```python
from build123d import *

# Parameters (mm, degrees)
SKETCH_3_W             = 131
SKETCH_3_H             = 80
EXTRUDE_3_DEPTH        = 5
SKETCH_4_W             = 119
SKETCH_4_H             = 80
EXTRUDE_4_DEPTH        = 6
FILLET_2_R             = 5
CHAMFER_1_SIZE         = 1
CUT_EXTRUDE_1_DEPTH    = 6
FILLET_3_R             = 5
CHAMFER_2_SIZE         = 1
SKETCH_6_R             = 2.2
CUT_EXTRUDE_2_DEPTH    = 11
HOLE_WIZARD_M3_1_D     = 2.5
HOLE_WIZARD_M3_1_DEPTH = 7.5
HOLE_WIZARD_M3_1_TIP   = 0.751075774
CHAMFER_3_SIZE         = 0.5


with BuildPart() as part:
    # 草图3 → 凸台-拉伸3 (new body)
    with BuildSketch(Plane.XY):
        with Locations((0, -51.5)):
            Rectangle(SKETCH_3_W, SKETCH_3_H)
    extrude(amount=EXTRUDE_3_DEPTH)

    # 草图4 → 凸台-拉伸4 (add)
    with BuildSketch(Plane.XY.offset(5)):
        with Locations((0, -51.5)):
            Rectangle(SKETCH_4_W, SKETCH_4_H)
    extrude(amount=-EXTRUDE_4_DEPTH)

    # 圆角2
    fillet_2_edges = [part.edges().sort_by_distance(p)[0] for p in [
        (-65.5, -11.5, 2.5),
        (65.5, -11.5, 2.5),
        (65.5, -91.5, 2.5),
        (-65.5, -91.5, 2.5),
    ]]
    fillet(fillet_2_edges, radius=FILLET_2_R)

    # 倒角1
    chamfer_1_edges = [part.edges().sort_by_distance(p)[0] for p in [
        (0, -11.5, 5),
        (65.5, -51.5, 5),
        (0, -91.5, 5),
        (-65.5, -51.5, 5),
        (64.035533906, -90.035533906, 5),
        (-64.035533906, -90.035533906, 5),
        (-64.035533906, -12.964466094, 5),
        (64.035533906, -12.964466094, 5),
    ]]
    chamfer(chamfer_1_edges, length=CHAMFER_1_SIZE)

    # 草图5 → 切除-拉伸1 (cut)
    with BuildSketch(Plane.XY.offset(5)):
        Polygon((-10.644021059, -51.5), (-54.5, -28.163791023), (-54.5, -74.836208978), align=None)
        Polygon((43.855978941, -22.5), (-43.855978941, -22.5), (0, -45.836208978), align=None)
        Polygon((54.5, -28.163791023), (10.644021059, -51.5), (54.5, -74.836208978), align=None)
        Polygon((43.855978941, -80.5), (0, -57.163791023), (-43.855978941, -80.5), align=None)
    extrude(amount=-CUT_EXTRUDE_1_DEPTH, mode=Mode.SUBTRACT)

    # 圆角3
    fillet_3_edges = [part.edges().sort_by_distance(p)[0] for p in [
        (10.644021059, -51.5, 2),
        (54.5, -28.163791023, 2),
        (54.5, -74.836208978, 2),
        (-43.855978941, -22.5, 2),
        (43.855978941, -22.5, 2),
        (0, -45.836208978, 2),
        (-43.855978941, -80.5, 2),
        (0, -57.163791023, 2),
        (43.855978941, -80.5, 2),
        (-54.5, -74.836208978, 2),
        (-54.5, -28.163791023, 2),
        (-10.644021059, -51.5, 2),
    ]]
    fillet(fillet_3_edges, radius=FILLET_3_R)

    # 倒角2
    chamfer_2_edges = [part.edges().sort_by_distance(p)[0] for p in [
        (33.045284631, -39.580061586, 5),
        (54.5, -51.5, 5),
        (33.045284631, -63.419938415, 5),
        (14.256439507, -38.250213644, 5),
        (-14.256439507, -38.250213644, 5),
        (0, -22.5, 5),
        (-33.045284631, -39.580061586, 5),
        (-33.045284631, -63.419938415, 5),
        (-54.5, -51.5, 5),
        (-14.256439507, -64.749786356, 5),
        (14.256439507, -64.749786356, 5),
        (0, -80.5, 5),
        (52.074521107, -32.201893935, 5),
        (52.074521107, -70.798106066, 5),
        (16.288042118, -51.5, 5),
        (0, -45.172417956, 5),
        (-28.666695849, -26.289632976, 5),
        (28.666695849, -26.289632976, 5),
        (-16.288042118, -51.5, 5),
        (-52.074521107, -70.798106066, 5),
        (-52.074521107, -32.201893935, 5),
        (0, -57.827582045, 5),
        (28.666695849, -76.710367025, 5),
        (-28.666695849, -76.710367025, 5),
    ]]
    chamfer(chamfer_2_edges, length=CHAMFER_2_SIZE)

    # 草图6 → 切除-拉伸2 (cut)
    with BuildSketch(Plane.XY.offset(5)):
        with Locations((62.5, -21.5)):
            Circle(SKETCH_6_R)
        with Locations((62.5, -31.5)):
            Circle(SKETCH_6_R)
        with Locations((62.5, -41.5)):
            Circle(SKETCH_6_R)
        with Locations((62.5, -51.5)):
            Circle(SKETCH_6_R)
        with Locations((62.5, -61.5)):
            Circle(SKETCH_6_R)
        with Locations((62.5, -71.5)):
            Circle(SKETCH_6_R)
        with Locations((62.5, -81.5)):
            Circle(SKETCH_6_R)
    cut_extrude_2 = extrude(amount=-CUT_EXTRUDE_2_DEPTH, mode=Mode.SUBTRACT)

    # 镜向1: 切除-拉伸2 across plane
    add(cut_extrude_2.mirror(Plane(origin=(0, 0, 0), x_dir=(0, 0, 1), z_dir=(1, 0, 0))), mode=Mode.SUBTRACT)

    # M3 螺纹孔1
    with Locations(Plane.XY.offset(5)):
        with Locations((-43.51, -20.75), (43.51, -20.75), (43.51, -80.29), (-43.51, -80.29)):
            Hole(HOLE_WIZARD_M3_1_D / 2, depth=HOLE_WIZARD_M3_1_DEPTH)
            with Locations((0, 0, -(HOLE_WIZARD_M3_1_DEPTH + HOLE_WIZARD_M3_1_TIP / 2))):  # 118° drill point
                Cone(0, HOLE_WIZARD_M3_1_D / 2, HOLE_WIZARD_M3_1_TIP, mode=Mode.SUBTRACT)

    # 倒角3
    chamfer_3_edges = [part.edges().sort_by_distance(p)[0] for p in [
        (33.045284631, -39.580061586, -1),
        (54.5, -51.5, -1),
        (33.045284631, -63.419938415, -1),
        (14.256439507, -38.250213644, -1),
        (-60, -11.5, 0),
        (-14.256439507, -38.250213644, -1),
        (0, -22.5, -1),
        (60, -91.5, 0),
        (-33.045284631, -39.580061586, -1),
        (-33.045284631, -63.419938415, -1),
        (-54.5, -51.5, -1),
        (-14.256439507, -64.749786356, -1),
        (14.256439507, -64.749786356, -1),
        (0, -80.5, -1),
        (52.074521107, -32.201893935, -1),
        (52.074521107, -70.798106066, -1),
        (16.288042118, -51.5, -1),
        (0, -45.172417956, -1),
        (-28.666695849, -26.289632976, -1),
        (28.666695849, -26.289632976, -1),
        (-16.288042118, -51.5, -1),
        (-52.074521107, -70.798106066, -1),
        (-52.074521107, -32.201893935, -1),
        (0, -57.827582045, -1),
        (28.666695849, -76.710367025, -1),
        (-28.666695849, -76.710367025, -1),
        (0, -91.5, -1),
        (0, -11.5, -1),
        (60, -11.5, 0),
        (65.5, -51.5, 0),
        (64.035533906, -90.035533906, 0),
        (64.035533906, -12.964466094, 0),
        (-65.5, -51.5, 0),
        (-60, -91.5, 0),
        (-64.035533906, -90.035533906, 0),
        (-64.035533906, -12.964466094, 0),
    ]]
    chamfer(chamfer_3_edges, length=CHAMFER_3_SIZE)


solid = part.part
```
The model under review builds one solid part; all positions refer to its coordinate system, in mm. A direction names the side the tool comes from. Coordinates: 2 decimals unless noted, no trailing zeros. Write each loop counter-clockwise with the first axis right and the second up, starting at its lowest first coordinate (ties: lowest second). Pieces come first, ordered by that corner, then holes.
1) The part is to be moulded in two halves that separate along X. For faces 4 (the face through (-52.228, -70.908, 4.174)), 5 (the face through (63.741, -89.814, 0.135)), say which applies: pulls with the +X half, pulls with the -X half, needs draft (parallel to the pull), parting line crosses it, or undercut.
2) Clearance check with flat-ended pins moving along their axes: pin 1 Ø4 at (x, y) = (-62.5, -81.5) entering from -Z; pin 2 Ø1.6 at (x, y) = (-61.5, -34.5) entering from -Z. State where each tip first meets the part, or that it passes through.
3) Machinability: for faces 1 (the face through (28.774, -76.835, -0.635)), 2 (the face through (14.66, -64.39, 4.51)), 3 (the face through (-33.2, -63.5, 1.8)), which of the approach directions +Z, -Z, +X, -X, +Y, -Y give a long, thin tool a straight path to every point of the face, cutting with its end or side? Answer none if there is none.
4) To check wall thickness, follow probe 1 along X at (y, z) = (-72.5, 3); probe 2 along X at (y, z) = (-21.5, 2.4); probe 3 along Y at (x, z) = (12.5, 1.5). State the ranges of each line that lie inside material, in increasing order.
5) We need section A-A on x = 34.5. State the section outline as (y, z) points.
6) We need section B-B on z = 3. Count the separate pieces of the cut face and the enclosed holes in it, then the cut area to 3 significant figures.
7) We need section C-C on x = -35. State the section outline as (y, z) points, then the cut area to 3 significant figures.
Answer list:
1. face 4: undercut
1. face 5: pulls with the +X half
2. pin 1: passes through
2. pin 2: stops at z = 0
3. face 1: -Z
3. face 2: +Z
3. face 3: +Z, -Z
4. probe 1: x = -65.5 to -64.46, -60.54 to -27.82, 27.82 to 60.54, 64.46 to 65.5
4. probe 2: x = -65.5 to -64.7, -60.3 to -44.51, -42.51 to 42.51, 44.51 to 60.3, 64.7 to 65.5
4. probe 3: y = -91.5 to -80.5, -63.82 to -39.18, -22.5 to -11.5
5. outline: (-91.5, -0.5) - (-91, -1) - (-64.76, -1) - (-64.19, -0.5) - (-64.19, 4) - (-65.33, 5) - (-90.5, 5) - (-91.5, 4) - close; (-38.81, -0.5) - (-38.24, -1) - (-12, -1) - (-11.5, -0.5) - (-11.5, 4) - (-12.5, 5) - (-37.67, 5) - (-38.81, 4) - close
6. separate pieces: 1
6. enclosed holes: 22
6. area: 6,510 mm2
7. outline: (-91.5, -0.5) - (-91, -1) - (-65.03, -1) - (-64.46, -0.5) - (-64.46, 4) - (-65.59, 5) - (-90.5, 5) - (-91.5, 4) - close; (-38.54, -0.5) - (-37.97, -1) - (-12, -1) - (-11.5, -0.5) - (-11.5, 4) - (-12.5, 5) - (-37.41, 5) - (-38.54, 4) - close
7. area: 322 mm2
